from build123d import *

# Parameters (mm, degrees)
SKETCH_BODY_R                       = 19
BODY_DEPTH                          = 20
SKETCH_CUT_BODY_W                   = 16
SKETCH_CUT_BODY_H                   = 6.627416998
REINFORCMENT_STRIP_REACH            = 36.641
CIRPATTERN_REINFORCMENT_STRIP_COUNT = 4
SKETCH_FIXING_HOLE_R                = 2.15
FIXING_HOLE_DEPTH                   = 35.641016151
CIRPATTERN_FIXING_HOLE_COUNT        = 4
BONE_DEPTH                          = 2
CIRPATTERN_BONE_COUNT               = 3
SKETCH_FIXING_PLATE_FAN_R           = 11.5
FIXING_PLATE_FAN_DEPTH              = 2
AIR_EXHAUST_DEPTH                   = 49.582404222


with BuildPart() as part:
    # Sketch-Body → Body (new body)
    with BuildSketch(Plane.XY):
        with BuildLine():
            Line((-16, -20), (16, -20))
            ThreePointArc((16, -20), (18.828427125, -18.828427125), (20, -16))
            Line((20, -16), (20, 16))
            ThreePointArc((20, 16), (18.828427125, 18.828427125), (16, 20))
            Line((16, 20), (-16, 20))
            ThreePointArc((-16, 20), (-18.828427125, 18.828427125), (-20, 16))
            Line((-20, 16), (-20, -16))
            ThreePointArc((-20, -16), (-18.828427125, -18.828427125), (-16, -20))
        make_face()
        Circle(SKETCH_BODY_R, mode=Mode.SUBTRACT)
    extrude(amount=BODY_DEPTH)

    # Sketch-Cut-Body → Cut-Body (revolve, cut)
    with BuildSketch(Plane(origin=(0, 0, 0), x_dir=(0, 0, -1), z_dir=(1, 0, 0)), mode=Mode.PRIVATE) as cut_body_sk:
        with Locations((-10, 23.313708499)):
            Rectangle(SKETCH_CUT_BODY_W, SKETCH_CUT_BODY_H)
    revolve(cut_body_sk.sketch.rotate(Axis((0, 0, 20), (0, 0, -1)), 180), axis=Axis((0, 0, 20), (0, 0, -1)), mode=Mode.SUBTRACT)

    # Sketch-Reinforcment-Strip → Reinforcment-Strip (add, up to next)
    with BuildSketch(Plane.XY, mode=Mode.PRIVATE) as reinforcment_strip_sk1:
        with BuildLine():
            Line((16.684833585, 11.027979336), (18.828427125, 13.171572875))
            ThreePointArc((18.828427125, 13.171572875), (18.828427125, 18.828427125), (13.171572875, 18.828427125))
            Line((13.171572875, 18.828427125), (11.027979336, 16.684833585))
            ThreePointArc((11.027979336, 16.684833585), (14.142135624, 14.142135624), (16.684833585, 11.027979336))
        make_face()
    reinforcment_strip_tool1 = extrude(reinforcment_strip_sk1.sketch, amount=REINFORCMENT_STRIP_REACH, mode=Mode.PRIVATE) - part.part
    reinforcment_strip = reinforcment_strip_tool1.solids().sort_by_distance((16.181232, 16.181232, 0))[0]
    add(reinforcment_strip)

    # CirPattern-Reinforcment-Strip: Reinforcment-Strip ×4 about axis
    cirpattern_reinforcment_strip_axis = Axis((0, 0, 0), (0, 0, 1))
    for i in range(1, CIRPATTERN_REINFORCMENT_STRIP_COUNT):
        add(reinforcment_strip.rotate(cirpattern_reinforcment_strip_axis, i * 360 / CIRPATTERN_REINFORCMENT_STRIP_COUNT))

    # Sketch-Fixing-Hole → Fixing-Hole (cut, through all)
    with BuildSketch(Plane.XY):
        with Locations((16, 16)):
            Circle(SKETCH_FIXING_HOLE_R)
    fixing_hole = extrude(amount=FIXING_HOLE_DEPTH, mode=Mode.SUBTRACT)

    # CirPattern-Fixing-Hole: Fixing-Hole ×4 about axis
    cirpattern_fixing_hole_axis = Axis((0, 0, 0), (0, 0, 1))
    for i in range(1, CIRPATTERN_FIXING_HOLE_COUNT):
        add(fixing_hole.rotate(cirpattern_fixing_hole_axis, i * 360 / CIRPATTERN_FIXING_HOLE_COUNT), mode=Mode.SUBTRACT)

    # Sketch-Bone → Bone (add)
    with BuildSketch(Plane.XY):
        with BuildLine():
            Line((-10.98406242, -3.405931994), (-15.423655551, -11.09553286))
            ThreePointArc((-15.423655551, -11.09553286), (-16.055816657, -10.159269239), (-16.631216794, -9.187090287))
            Line((-16.631216794, -9.187090287), (-11.496264484, -0.293091992))
            ThreePointArc((-11.496264484, -0.293091992), (-11.347410174, -1.867158898), (-10.98406242, -3.405931994))
        make_face()
    bone = extrude(amount=BONE_DEPTH)

    # CirPattern-Bone: Bone ×3 about axis
    cirpattern_bone_axis = Axis((0, 0, 0), (0, 0, 1))
    for i in range(1, CIRPATTERN_BONE_COUNT):
        add(bone.rotate(cirpattern_bone_axis, i * 360 / CIRPATTERN_BONE_COUNT))

    # Sketch-Fixing-Plate-Fan → Fixing-Plate-Fan (add)
    with BuildSketch(Plane.XY):
        Circle(SKETCH_FIXING_PLATE_FAN_R)
    extrude(amount=FIXING_PLATE_FAN_DEPTH)

    # Sketch2 → Air-Exhaust (cut, through all)
    with BuildSketch(Plane(origin=(0, 19.5, 0), x_dir=(-1, 0, 0), z_dir=(0, 1, 0))):
        Polygon((-1.750518846, 7.5), (0, 5), (1.750518846, 7.5), (0.881634904, 7.5), (0.881634904, 10), (-0.881634904, 10), (-0.881634904, 7.5), align=None)
    extrude(amount=AIR_EXHAUST_DEPTH, mode=Mode.SUBTRACT)


solid = part.part
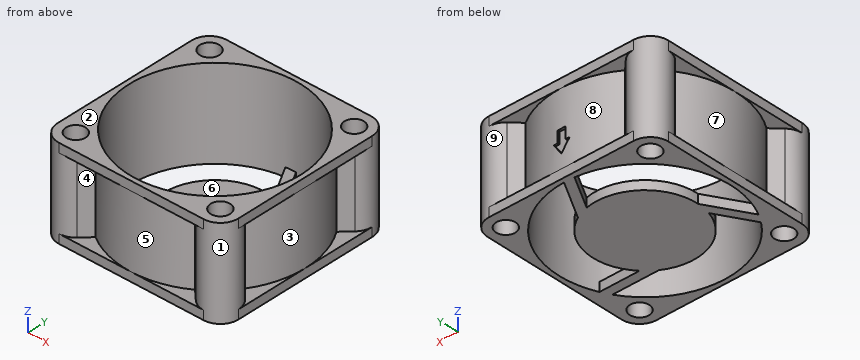
Part model, mm, in its own coordinate system. Face numbers are marked on the shaded views. A direction names the side the tool comes from. Coordinates: 2 decimals unless noted, no trailing zeros. Order: outer loops, then holes, each group sorted by start corner. A loop starts at its lowest first (then second) coordinate and runs counter-clockwise, first axis right, second up. Notation, with made-up numbers: M 25,88.25 L 38,88.25 A13 ccw 38,104.25 Z; hole C 63,-19 d1. An arc over 180 degrees is marked long. One line per question, with ' | ' between items.
Q1. Two-plate mould, pull along Y, no slides. Class the marked faces 1, 2, 3 and 4: +Y half, -Y half, draft (parallel to the pull), parting line (faces both ways), or undercut.
A:
face 1: undercut | face 2: draft | face 3: undercut | face 4: -Y half
Q2. Slice it at A-A (z = 8.75). Give the cut face in (x, y).
A:
outline: M -18.83,-13.17 A4 ccw -13.17,-18.83 L -11.03,-16.68 A20 ccw 11.03,-16.68 L 13.17,-18.83 A4 ccw 18.83,-13.17 L 16.68,-11.03 A20 ccw 16.68,11.03 L 18.83,13.17 A4 ccw 13.17,18.83 L 11.03,16.68 A20 ccw 0.88,19.98 L 0.88,19.5 L -0.88,19.5 L -0.88,19.98 A20 ccw -11.03,16.68 L -13.17,18.83 A4 ccw -18.83,13.17 L -16.68,11.03 A20 ccw -16.68,-11.03 Z; hole C 0,0 d38; hole C -16,-16 d4.3; hole C -16,16 d4.3; hole C 16,-16 d4.3; hole C 16,16 d4.3
Q3. Slice it at B-B (y = -10.5). Give the cut face in (x, z), and give its area (3 significant figures).
A:
outline: M -20,0 L -15.08,0 L -15.08,2 L -15.84,2 L -15.84,20 L -20,20 L -20,18 L -17.02,18 L -17.02,2 L -20,2 Z; M -4.69,0 L 4.69,0 L 4.69,2 L -4.69,2 Z; M 15.84,0 L 20,0 L 20,2 L 17.02,2 L 17.02,18 L 20,18 L 20,20 L 15.84,20 Z | area: 91.6 mm^2
Q4. Pin check, flat tips, straight feed: P1, Ø4, axis at x = 10.5, y = -12, coming from the +Z side; P2, Ø4, axis at x = 0.5, z = 6.5, coming from the +Y side; P3, Ø4, axis at x = -12, y = -2.5, coming from the +Z side; P4, Ø2, axis at x = 2, z = 14, coming from the -Y side (3 decimals). Stop position of each tip, or through.
A:
P1: passes through | P2: stops at y = 20 | P3: stops at z = 2 | P4: stops at y = -19.975
Q5. Slice it at D-D (z = 12.75). Give the cut face in (x, y), and give its area (3 significant figures).
A:
outline: M -18.83,-13.17 A4 ccw -13.17,-18.83 L -11.03,-16.68 A20 ccw 11.03,-16.68 L 13.17,-18.83 A4 ccw 18.83,-13.17 L 16.68,-11.03 A20 ccw 16.68,11.03 L 18.83,13.17 A4 ccw 13.17,18.83 L 11.03,16.68 A20 ccw -11.03,16.68 L -13.17,18.83 A4 ccw -18.83,13.17 L -16.68,11.03 A20 ccw -16.68,-11.03 Z; hole C 0,0 d38; hole C -16,-16 d4.3; hole C -16,16 d4.3; hole C 16,-16 d4.3; hole C 16,16 d4.3 | area: 253 mm^2
Q6. 3-axis set-ups, long thin cutter, end or side, ignore diameter. For the marked faces 5, 6, 7, 8 and 9: which of +Z, -Z, +X, -X, +Y, -Y reach the whole face in a straight line?
A:
face 5: -Y | face 6: +Z | face 7: -X | face 8: +Y | face 9: none
Q7. Drill centre lines: line 1 (Y direction, x = 16, z = 8.25); line 2 (X direction, y = 14.5, z = 1.75). Where is each one in solid material? Low to high.
A:
line 1: y = -20 to -18.15, -13.85 to -10.25, 10.25 to 13.85, 18.15 to 20 | line 2: x = -20 to -17.54, -14.46 to -12.28, 0.65 to 2.96, 12.28 to 14.46, 17.54 to 20
Q8. Slice it at C-C (x = -9). Give the cut face in (y, z).
A:
outline: M -20,0 L -16.73,0 L -16.73,20 L -20,20 L -20,18 L -17.86,18 L -17.86,2 L -20,2 Z; M -7.16,0 L 7.16,0 L 7.16,2 L -7.16,2 Z; M 16.73,0 L 20,0 L 20,2 L 17.86,2 L 17.86,18 L 20,18 L 20,20 L 16.73,20 Z
